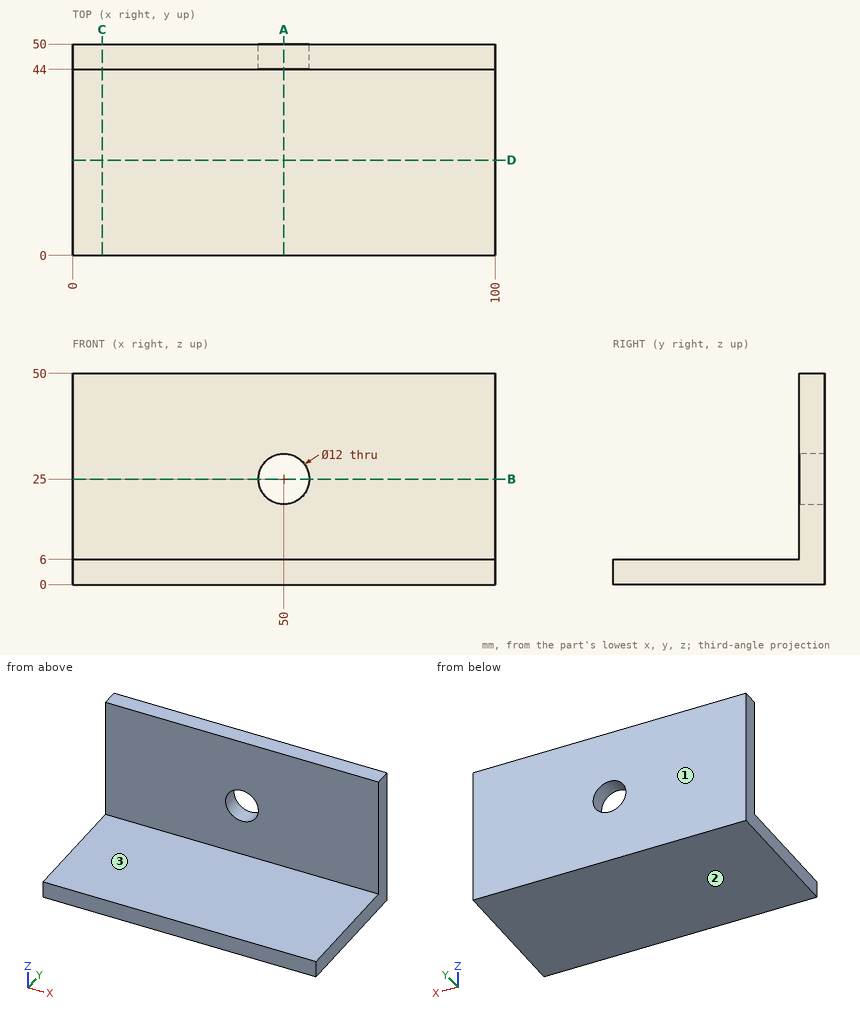
Design review of the part shown in the three views and the two pictorial views. Dimensions are in mm from the part's minimum x, y and z. Round coordinates to 2 decimals unless told otherwise and drop trailing zeros. Order: outer loops, then holes, each group sorted by start corner. A loop starts at its lowest first (then second) coordinate and runs counter-clockwise, first axis right, second up.
Item 1: Add section C-C, the plane x = 7. State the section outline as (y, z) points.
Working result:
outline: (0, 0) - (50, 0) - (50, 50) - (44, 50) - (44, 6) - (0, 6) - close
Item 2: To check wall thickness, follow probe 1 along X at (y, z) = (46.7, 25); probe 2 along Z at (x, y) = (70, 29); probe 3 along Y at (x, z) = (29.5, 20.5). State the ranges of each line that lie inside material, in increasing order.
Working result:
probe 1: x = 0 to 44, 56 to 100
probe 2: z = 0 to 6
probe 3: y = 44 to 50
Item 3: Add section A-A, the plane x = 50. State the section outline as (y, z) points, and give its area (3 significant figures).
Working result:
outline: (0, 0) - (50, 0) - (50, 19) - (44, 19) - (44, 6) - (0, 6) - close; (44, 31) - (50, 31) - (50, 50) - (44, 50) - close
area: 492 mm2
Item 4: Draft analysis for pull direction Z (two halves, no side actions). For the marked faces 1, 2 and 3, state which applies: released by +Z, released by -Z, zero draft, split by the parting line, or undercut.
Working result:
face 1: zero draft
face 2: released by -Z
face 3: released by +Z
Item 5: Add section B-B, the plane z = 25. State the section outline as (x, y) points.
Working result:
outline: (0, 44) - (44, 44) - (44, 50) - (0, 50) - close; (56, 44) - (100, 44) - (100, 50) - (56, 50) - close
Item 6: Add section D-D, the plane y = 22.5. State the section outline as (x, z) points.
Working result:
outline: (0, 0) - (100, 0) - (100, 6) - (0, 6) - close
Item 7: For pin 1 (8 mm diameter, centred on x = 89, y = 28.5, fed in from +Z); pin 2 (19 mm diameter, centred on x = 50, z = 25, fed in from -Y); pin 3 (12 mm diameter, centred on x = 38, z = 8, fed in from -Y), all flat-tipped, find the tip position at first contact; note any pin that passes through.
Working result:
pin 1: stops at z = 6
pin 2: stops at y = 44
pin 3: stops at y = 0
